Study the drawing (mm; zero at the part's minimum x, y, z) and answer. Coordinates: 2 decimals unless noted, no trailing zeros. Order: outer loops, then holes, each group sorted by start corner. A loop starts at its lowest first (then second) coordinate and runs counter-clockwise, first axis right, second up.
1. Find the intervals of material crossed by probe 1 along X at (y, z) = (11.5, 2.55); probe 2 along X at (y, z) = (42, 1.55); probe 3 along Y at (x, z) = (9.5, 0.9), in increasing order.
2. The part is cut by section B-B, the plane y = 34.5. Give the vertices of the cut face in (x, z), then the cut area to 3 significant figures.
3. The part is cut by section D-D, the plane x = 39. Give the vertices of the cut face in (y, z), then the cut area to 3 significant figures.
4. The part is cut by section A-A, the plane x = 10. Give the vertices of the cut face in (y, z), then the cut area to 3 significant figures.
5. The part is cut by section C-C, the plane z = 1.55. Give the vertices of the cut face in (x, y).
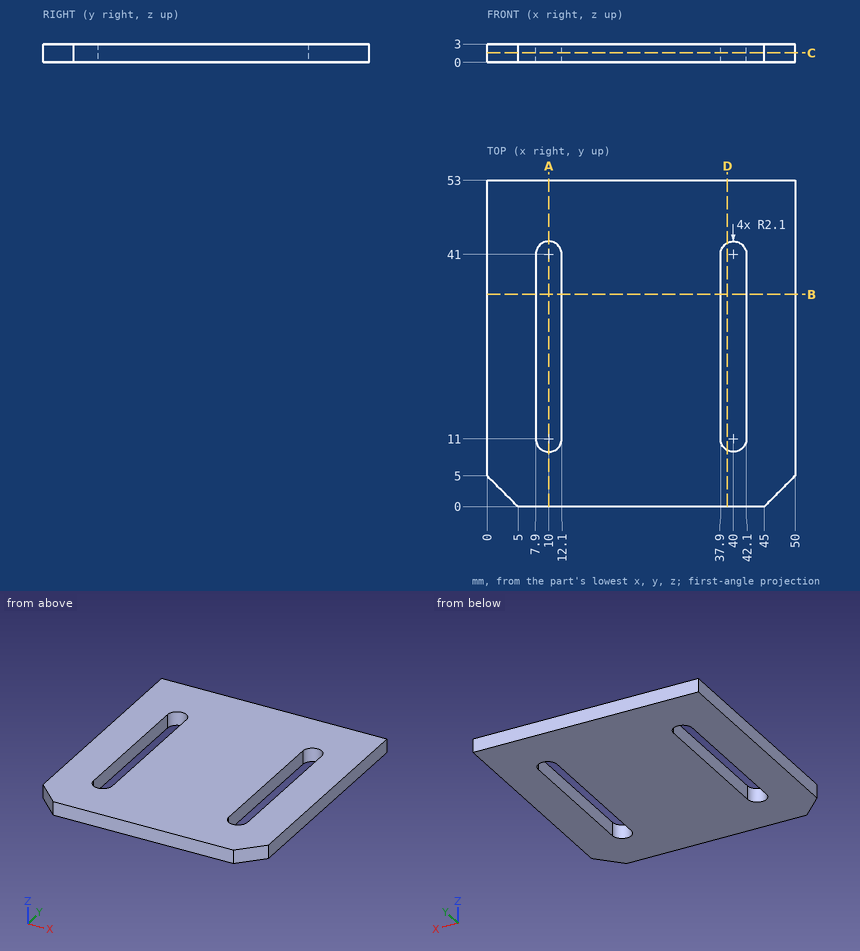
Geometry says:
1. probe 1: x = 0 to 7.9, 12.1 to 37.9, 42.1 to 50
1. probe 2: x = 0 to 8.15, 11.85 to 38.15, 41.85 to 50
1. probe 3: y = 0 to 8.96, 43.04 to 53
2. outline: (0, 0) - (7.9, 0) - (7.9, 3) - (0, 3) - close; (12.1, 0) - (37.9, 0) - (37.9, 3) - (12.1, 3) - close; (42.1, 0) - (50, 0) - (50, 3) - (42.1, 3) - close
2. area: 125 mm2
3. outline: (0, 0) - (9.15, 0) - (9.15, 3) - (0, 3) - close; (42.85, 0) - (53, 0) - (53, 3) - (42.85, 3) - close
3. area: 57.9 mm2
4. outline: (0, 0) - (8.9, 0) - (8.9, 3) - (0, 3) - close; (43.1, 0) - (53, 0) - (53, 3) - (43.1, 3) - close
4. area: 56.4 mm2
5. outline: (0, 5) - (5, 0) - (45, 0) - (50, 5) - (50, 53) - (0, 53) - close; hole (7.9, 11) arc R2.1 ccw to (12.1, 11) - (12.1, 41) arc R2.1 ccw to (7.9, 41) - close; hole (37.9, 11) arc R2.1 ccw to (42.1, 11) - (42.1, 41) arc R2.1 ccw to (37.9, 41) - close
